For this review, take the finished solid that the model builds, in its own axes (mm). Face numbers are marked on the shaded views. A direction names the side the tool comes from. Give positions to 0.01 mm unless a question says otherwise; leave off trailing zeros. Loops run counter-clockwise (first coordinate to the right, second up) from the corner with the lowest first, then second, coordinate; pieces in that order, holes last.
```python
from build123d import *

# Parameters (mm, degrees)
ESQUISSE1_R                = 23.5
BOSS_EXTRU_1_DEPTH         = 10
ENL_V_MAT_EXTRU_1_DEPTH    = 10
ESQUISSE4_R                = 16.5
ENL_V_MAT_EXTRU_2_DEPTH    = 1
R_P_TITION_LIN_AIRE1_COUNT = 2
R_P_TITION_LIN_AIRE1_PITCH = 9


with BuildPart() as part:
    # Esquisse1 → Boss.-Extru.1 (new body)
    with BuildSketch(Plane.XY):
        Circle(ESQUISSE1_R)
    extrude(amount=BOSS_EXTRU_1_DEPTH)

    # Esquisse3 → Enlèv. mat.-Extru.1 (cut)
    with BuildSketch(Plane.XY.offset(10)):
        Polygon((-7.501301233, 0), (-3.749717926, 6.494701961), (3.75, 6.495190528), (7.5, 0), align=None)
    enl_v_mat_extru_1 = extrude(amount=-ENL_V_MAT_EXTRU_1_DEPTH, mode=Mode.SUBTRACT)

    # Symétrie1: Enlèv. mat.-Extru.1 across plane
    add(enl_v_mat_extru_1.mirror(Plane.ZX), mode=Mode.SUBTRACT)

    # Esquisse4 → Enlèv. mat.-Extru.2 (cut)
    with BuildSketch(Plane.XY.offset(10)):
        Circle(ESQUISSE4_R)
    enl_v_mat_extru_2 = extrude(amount=-ENL_V_MAT_EXTRU_2_DEPTH, mode=Mode.SUBTRACT)

    # Répétition linéaire1: Enlèv. mat.-Extru.2 ×2
    with Locations(*[(0, 0, -i * R_P_TITION_LIN_AIRE1_PITCH) for i in range(1, R_P_TITION_LIN_AIRE1_COUNT)]):
        add(enl_v_mat_extru_2, mode=Mode.SUBTRACT)


solid = part.part
```
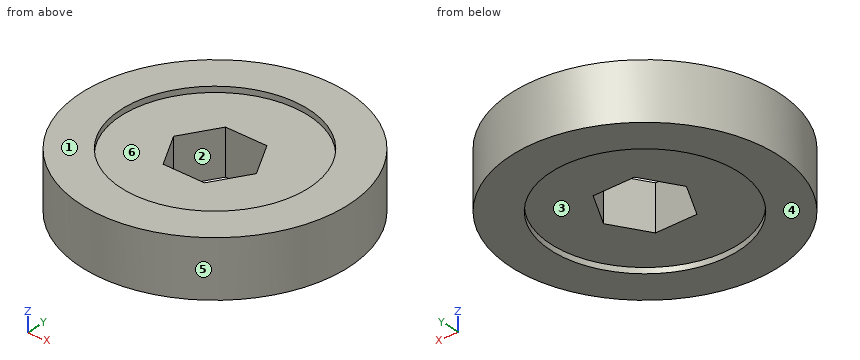
Item 1: Take a section at B-B on x = 0. Give the boundary of the cut face in (y, z).
Answer:
outline: (-23.5, 0) - (-16.5, 0) - (-16.5, 1) - (-6.49, 1) - (-6.49, 9) - (-16.5, 9) - (-16.5, 10) - (-23.5, 10) - close; (6.49, 1) - (16.5, 1) - (16.5, 0) - (23.5, 0) - (23.5, 10) - (16.5, 10) - (16.5, 9) - (6.49, 9) - close
Item 2: Clearance check with flat-ended pins moving along their axes: pin 1 Ø2 at (x, z) = (1.5, 6) entering from -Y; pin 2 Ø6 at (x, z) = (-0.5, 6.5) entering from +Y; pin 3 Ø4 at (y, z) = (-11, 8) entering from -X. State where each tip first meets the part, or that it passes through.
Answer:
pin 1: stops at y = -23.49
pin 2: stops at y = 23.5
pin 3: stops at x = -21.71
Item 3: Take a section at A-A on z = 6.75. Give the boundary of the cut face in (x, y).
Answer:
outline: circle Ø47 at (0, 0); hole (-7.5, 0) - (-3.75, -6.49) - (3.75, -6.5) - (7.5, 0) - (3.75, 6.5) - (-3.75, 6.49) - close
Item 4: Tool access review of the marked faces 1, 2 and 3: name each direction out of +Z, -Z, +X, -X, +Y, -Y from which nothing blocks a thin tool from reaching the whole face with its end or side.
Answer:
face 1: +Z, +X, -X, +Y, -Y
face 2: +Z, -Z
face 3: -Z
Item 5: The part is to be moulded in two halves that separate along Y. For the marked faces 4, 5 and 6, say which applies: released by +Y, released by -Y, zero draft, split by the parting line, or undercut.
Answer:
face 4: zero draft
face 5: split by the parting line
face 6: undercut
Item 6: For L1, parallel to Y at x = 0, z = 0.25; L2, parallel to Y at x = 0, z = 4.5; L3, parallel to X at y = -4.5, z = 6.75, list the stretches that pass through material, from the lowest coordinate up.
Answer:
L1: y = -23.5 to -16.5, 16.5 to 23.5
L2: y = -23.5 to -6.49, 6.49 to 23.5
L3: x = -23.07 to -4.9, 4.9 to 23.07
Item 7: Take a section at C-C on y = -4. Give the boundary of the cut face in (x, z).
Answer:
outline: (-23.16, 0) - (-16.01, 0) - (-16.01, 1) - (-5.19, 1) - (-5.19, 9) - (-16.01, 9) - (-16.01, 10) - (-23.16, 10) - close; (5.19, 1) - (16.01, 1) - (16.01, 0) - (23.16, 0) - (23.16, 10) - (16.01, 10) - (16.01, 9) - (5.19, 9) - close
Item 8: Take a section at D-D on x = 12. Give the boundary of the cut face in (y, z), and give its area (3 significant figures).
Answer:
outline: (-20.21, 0) - (-11.32, 0) - (-11.32, 1) - (11.32, 1) - (11.32, 0) - (20.21, 0) - (20.21, 10) - (11.32, 10) - (11.32, 9) - (-11.32, 9) - (-11.32, 10) - (-20.21, 10) - close
area: 359 mm2
